Design review of the part built by this model. Coordinates are the model's own, in mm. Give positions to 0.01 mm unless a question says otherwise; leave off trailing zeros. Write each loop counter-clockwise with the first axis right and the second up, starting at its lowest first coordinate (ties: lowest second). Pieces come first, ordered by that corner, then holes. Notation, with made-up numbers: (-24.5, 65) -> (27.5, 65) arc R6 cw to (27.5, 76) -> close; hole circle Ø5 at (29, 42.5). An arc over 180 degrees is marked (long way). Use CSV: the item, a comma, the result in double quotes.
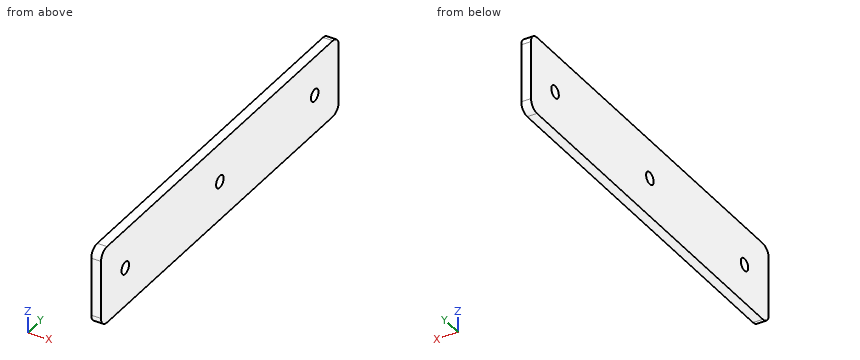
```python
from build123d import *

# Parameters (mm, degrees)
F0_R     = 4
F1_DEPTH = 6.35


with BuildPart() as f1:
    # F0 (on Right) → F1 (new body)
    with BuildSketch(Plane.YZ):
        with BuildLine():
            Line((120.65, 25.4), (-120.65, 25.4))
            ThreePointArc((-120.65, 25.4), (-125.140128, 23.540128), (-127, 19.05))
            Line((-127, 19.05), (-127, 0))
            Line((-127, 0), (-127, -19.05))
            ThreePointArc((-127, -19.05), (-125.140128, -23.540128), (-120.65, -25.4))
            Line((-120.65, -25.4), (120.65, -25.4))
            ThreePointArc((120.65, -25.4), (125.140128, -23.540128), (127, -19.05))
            Line((127, -19.05), (127, 0))
            Line((127, 0), (127, 19.05))
            ThreePointArc((127, 19.05), (125.140128, 23.540128), (120.65, 25.4))
        make_face()
        with BuildLine():
            ThreePointArc((-97.123065, 0), (-101.123065, -4), (-105.123065, 0))
            ThreePointArc((-105.123065, 0), (-101.123065, 4), (-97.123065, 0))
        make_face(mode=Mode.SUBTRACT)
        Circle(F0_R, mode=Mode.SUBTRACT)
        with Locations((101.316608, 0)):
            Circle(F0_R, mode=Mode.SUBTRACT)
    extrude(amount=F1_DEPTH)


solid = f1.part
```
(1) For line 1 along Z through (x, y) = (4.5, 101); line 2 along Y through (x, z) = (2.25, -23), list the stretches that pass through material, from the lowest coordinate up. Write a range as [from, to].
Established:
line 1,"z = [-25.4, -3.99], [3.99, 25.4]"
line 2,"y = [-125.62, 125.62]"
(2) Take a section at A-A (y = 0). Write out the cut boundary in (x, z), then the cut area to 3 significant figures.
Established:
outline,"(0, -25.4) -> (6.35, -25.4) -> (6.35, -4) -> (0, -4) -> close; (0, 4) -> (6.35, 4) -> (6.35, 25.4) -> (0, 25.4) -> close"
area,"272 mm2"
(3) Take a section at B-B (z = 0). Write out the cut boundary in (x, y), then the cut area to 3 significant figures.
Established:
outline,"(0, -127) -> (6.35, -127) -> (6.35, -105.12) -> (0, -105.12) -> close; (0, -97.12) -> (6.35, -97.12) -> (6.35, -4) -> (0, -4) -> close; (0, 4) -> (6.35, 4) -> (6.35, 97.32) -> (0, 97.32) -> close; (0, 105.32) -> (6.35, 105.32) -> (6.35, 127) -> (0, 127) -> close"
area,"1,460 mm2"
